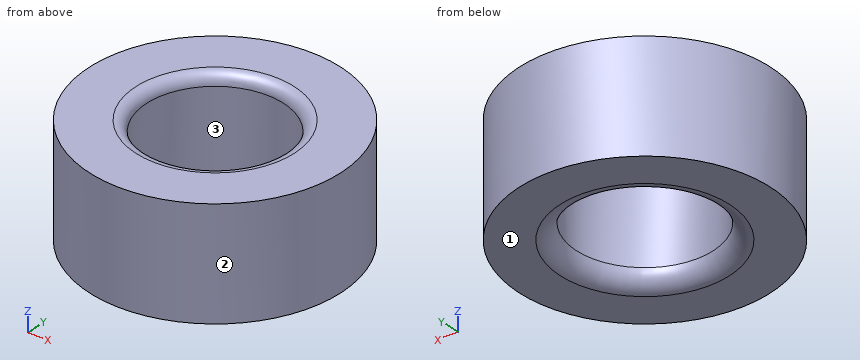
from build123d import *

# Parameters (mm, degrees)
F0_R     = 58.504478
F0_R_2   = 31.821293
F1_DEPTH = 50.8
F2_R     = 5.08
F3_R     = 7.62


with BuildPart() as f1:
    # F0 (on Top) → F1 (new body)
    with BuildSketch(Plane.XY):
        Circle(F0_R)
        Circle(F0_R_2, mode=Mode.SUBTRACT)
    extrude(amount=F1_DEPTH)

    # F2
    f2_edges = [f1.edges().sort_by_distance(p)[0] for p in [
        (-31.821293, 0, 50.8),
    ]]
    fillet(f2_edges, radius=F2_R)

    # F3
    f3_edges = [f1.edges().sort_by_distance(p)[0] for p in [
        (-31.821293, 0, 0),
    ]]
    fillet(f3_edges, radius=F3_R)


solid = f1.part
The model under review builds one solid part; all positions refer to its coordinate system, in mm. Face numbers are marked on the shaded views. Round coordinates to 2 decimals unless told otherwise and drop trailing zeros. Write each loop counter-clockwise with the first axis right and the second up, starting at its lowest first coordinate (ties: lowest second). Pieces come first, ordered by that corner, then holes. Notation, with made-up numbers: (-25.5, 18) - (-16.5, 18) arc R14 cw to (-16.5, 40) - close; hole circle Ø4 at (51, 6). An arc over 180 degrees is marked (long way). One line per item, written item: value. Start each with the question number.
1. Consider section A-A on x = 0. Write out the cut boundary in (y, z).
2. Consider section D-D on y = -45.5. Write out the cut boundary in (x, z).
3. To check wall thickness, follow L1, parallel to Y at x = 0, z = 20.5; L2, parallel to X at y = 21.5, z = 19.5; L3, parallel to Y at x = -17.5, z = 35.5. State the ranges of each line that lie inside material, in increasing order. Write a range as from..to.
4. Consider section C-C on z = 43.5. Write out the cut boundary in (x, y).
5. The part is to be moulded in two halves that separate along Y. For the marked faces 1, 2 and 3, say which applies: released by +Y, released by -Y, zero draft, split by the parting line, or undercut.
6. Clearance check with flat-ended pins moving along their axes: P1, Ø3, axis at x = -27.5, y = -32.5, coming from the -Z side; P2, Ø2, axis at y = 21, z = 15.5, coming from the -X side; P3, Ø5, axis at x = 22.5, y = 24.5, coming from the +Z side; P4, Ø5, axis at x = 1.5, z = 22.5, coming from the -Y side. State where each tip first meets the part, or that it passes through.
Checks:
1. outline: (-58.5, 0) - (-39.44, 0) arc R7.62 ccw to (-31.82, 7.62) - (-31.82, 45.72) arc R5.08 ccw to (-36.9, 50.8) - (-58.5, 50.8) - close; (31.82, 7.62) arc R7.62 ccw to (39.44, 0) - (58.5, 0) - (58.5, 50.8) - (36.9, 50.8) arc R5.08 ccw to (31.82, 45.72) - close
2. outline: (-36.78, 0) - (36.78, 0) - (36.78, 50.8) - (-36.78, 50.8) - close
3. L1: y = -58.5..-31.82, 31.82..58.5
3. L2: x = -54.41..-23.46, 23.46..54.41
3. L3: y = -55.83..-26.58, 26.58..55.83
4. outline: circle Ø117.01 at (0, 0); hole circle Ø63.64 at (0, 0)
5. face 1: zero draft
5. face 2: split by the parting line
5. face 3: undercut
6. P1: stops at z = 0
6. P2: stops at x = -54.98
6. P3: stops at z = 50.67
6. P4: stops at y = -58.5
